Source: CAD feature listing. Evaluate the final solid. Frame: model axes, mm. A direction names the side the tool comes from. Coordinates: 2 decimals unless noted, no trailing zeros. Write each loop counter-clockwise with the first axis right and the second up, starting at its lowest first coordinate (ties: lowest second). Pieces come first, ordered by that corner, then holes. Notation, with made-up numbers: M 31,73 L 59,73 A31 ccw 59,108 Z; hole C -1,-22 d11. An arc over 180 degrees is marked long. One line per item, written item: value. Start each with the question number.
Item 1: Ray query, L1, parallel to Z at x = 239, y = 15.5; L2, parallel to X at y = -15, z = 21; L3, parallel to Y at x = 143.5, z = 80.5. Return the intervals inside material, ascending. Write a range as from..to.
Item 2: Set-up query: faces 4 (the flat face through (148, 32, 148)), 5 (the flat face through (-129.96, -67.15, 62.12)). Return all of +Z, -Z, +X, -X, +Y, -Y with unobstructed straight access to the full face (end or side cutting, diameter ignored); none if empty.
Item 3: Mould query, pull axis Z, two halves, no side actions, for faces 1 (the cylindrical face through (153.58, -9.406, 180.045)), 2 (the flat face through (148, 32, 213)), 3 (the flat face through (-44, 1, 8)). Classes: released by +Z, released by -Z, zero draft, split by the parting line, or undercut.
Item 4: Cut plane A-A, the plane z = 56. Output: boundary loops of the cut face in (x, y).
Item 5: Pin query (flat end, axial travel): P1, Ø12, axis at y = 35.5, z = 176, coming from the +X side; P2, Ø1, axis at y = -16.5, z = 80, coming from the +X side; P3, Ø5, axis at y = 0, z = 142.5, coming from the +X side; P4, Ø18, axis at x = 282, y = 0, coming from the +Z side. Return the tip coordinate at first contact, or that it passes through.
Item 6: Cut plane C-C, the plane x = 114. Output: boundary loops of the cut face in (y, z).
Item 7: Cut plane D-D, the plane x = 0. Output: boundary loops of the cut face in (y, z), then the cut area to 3 significant figures.
Item 8: Cut plane B-B, the plane x = 251. Output: boundary loops of the cut face in (y, z), then the cut area to 3 significant figures.
```python
from build123d import *

# Parameters (mm, degrees)
EXTRUSION1_DEPTH             = 126
ESQUISSE2_W                  = 110
ESQUISSE2_H                  = 140
ENL_V_MAT_EXTRU_1_DEPTH      = 200
ENL_V_MAT_EXTRU_2_DEPTH      = 55
ENL_V_MAT_EXTRU_2_DEPTH_BACK = 55
ESQUISSE6_OUTSIDE_W          = 705.578
ESQUISSE6_OUTSIDE_H          = 273.578
ESQUISSE8_R                  = 20
EXTRUSION2_DEPTH             = 85
ESQUISSE9_R                  = 25
EXTRUSION3_DEPTH             = 65
ESQUISSE10_R                 = 20
EXTRUSION4_DEPTH             = 20
ESQUISSE11_R                 = 10
ENL_V_MAT_EXTRU_3_DEPTH      = 362.007271395
ESQUISSE12_R                 = 10
ENL_V_MAT_EXTRU_4_DEPTH      = 362.007271395


with BuildPart() as part:
    # Esquisse1 → Extrusion1 (new body)
    with BuildSketch(Plane.XY):
        with BuildLine():
            Line((-251, 60), (-251, -60))
            Line((-251, -60), (-5.478634649, -74.5))
            Line((-5.478634649, -74.5), (286.372947888, -47.800390446))
            ThreePointArc((286.372947888, -47.800390446), (330, 0), (286.372947888, 47.800390446))
            Line((286.372947888, 47.800390446), (-5.478634649, 74.5))
            Line((-5.478634649, 74.5), (-251, 60))
        make_face()
    extrude(amount=EXTRUSION1_DEPTH)

    # Esquisse2 → Enlèv. mat.-Extru.1 (cut)
    with BuildSketch(Plane(origin=(158, 0, 0), x_dir=(0, 0, -1), z_dir=(1, 0, 0))):
        with Locations((-63, -30)):
            Rectangle(ESQUISSE2_W, ESQUISSE2_H)
    extrude(amount=ENL_V_MAT_EXTRU_1_DEPTH, mode=Mode.SUBTRACT)

    # Esquisse6 outside → Enlèv. mat.-Extru.2 (cut, two sides: drawn at the far end of the back side and taken through both)
    # profile 1 of 2: a face of its own
    with BuildSketch(Plane.XY.offset(63).offset(-ENL_V_MAT_EXTRU_2_DEPTH_BACK)):
        with Locations((39.5, 0)):
            Rectangle(ESQUISSE6_OUTSIDE_W, ESQUISSE6_OUTSIDE_H)
        Polygon((-251, 60), (-251, -60), (-5.478634649, -74.5), (158, -59.544399357), (158, 59.544399357), (-5.478634649, 74.5), align=None, mode=Mode.SUBTRACT)
    # profile 2 of 2: a face of its own
    with BuildSketch(Plane.XY.offset(63).offset(-ENL_V_MAT_EXTRU_2_DEPTH_BACK)):
        Polygon((152, 54.068245078), (152, -54.068245078), (-5.575624206, -68.483817558), (-245, -54.343893548), (-245, 54.343893548), (-5.575624206, 68.483817558), align=None)
    extrude(amount=ENL_V_MAT_EXTRU_2_DEPTH + ENL_V_MAT_EXTRU_2_DEPTH_BACK, mode=Mode.SUBTRACT)

    # Esquisse8 → Extrusion2 (add)
    with BuildSketch(Plane.XY.offset(63)):
        with Locations((159, 15)):
            Circle(ESQUISSE8_R)
    extrude(amount=EXTRUSION2_DEPTH)

    # Esquisse9 → Extrusion3 (add)
    with BuildSketch(Plane.XY.offset(148)):
        with Locations((159, 15)):
            Circle(ESQUISSE9_R)
    extrude(amount=EXTRUSION3_DEPTH)

    # Esquisse10 → Extrusion4 (add)
    with BuildSketch(Plane.XY.offset(213)):
        with Locations((159, 15)):
            Circle(ESQUISSE10_R)
    extrude(amount=EXTRUSION4_DEPTH)

    # Esquisse11 → Enlèv. mat.-Extru.3 (cut, through all)
    with BuildSketch(Plane.XY.offset(126)):
        with Locations((282, 0)):
            Circle(ESQUISSE11_R)
    extrude(amount=-ENL_V_MAT_EXTRU_3_DEPTH, mode=Mode.SUBTRACT)

    # Esquisse12 → Enlèv. mat.-Extru.4 (cut, through all)
    with BuildSketch(Plane.XY.offset(126)):
        Circle(ESQUISSE12_R)
    extrude(amount=-ENL_V_MAT_EXTRU_4_DEPTH, mode=Mode.SUBTRACT)


solid = part.part
```
From the geometry:
1. L1: z = 0..8, 118..126
1. L2: x = -251..-245, 152..158
1. L3: y = -60.87..-54.85, 2.36..27.64, 54.85..60.87
2. face 4: none
2. face 5: +Z, -Z, -X, -Y
3. face 1: zero draft
3. face 2: released by +Z
3. face 3: undercut
4. outline: M -251,-60 L -5.48,-74.5 L 158,-59.54 L 158,59.54 L -5.48,74.5 L -251,60 Z; hole M -245,-54.34 L -5.58,-68.48 L 152,-54.07 L 152,54.07 L -5.58,68.48 L -245,54.34 Z
5. P1: stops at x = 179.37
5. P2: stops at x = 158
5. P3: stops at x = 174.61
5. P4: passes through
6. outline: M -63.57,0 L 63.57,0 L 63.57,126 L -63.57,126 Z; hole M -57.54,8 L 57.54,8 L 57.54,118 L -57.54,118 Z
7. outline: M -74,0 L -10,0 L -10,8 L -67.97,8 L -67.97,118 L -10,118 L -10,126 L -74,126 Z; M 10,0 L 74,0 L 74,126 L 10,126 L 10,118 L 67.97,118 L 67.97,8 L 10,8 Z
7. area: 3,370 mm²
8. outline: M -51.04,0 L 51.04,0 L 51.04,8 L -51.04,8 Z; M -51.04,118 L 51.04,118 L 51.04,126 L -51.04,126 Z
8. area: 1,630 mm²
